Design review of the part built by this model. Coordinates are the model's own, in mm. A direction names the side the tool comes from. Give positions to 0.01 mm unless a question says otherwise; leave off trailing zeros. Loops run counter-clockwise (first coordinate to the right, second up) from the corner with the lowest first, then second, coordinate; pieces in that order, holes last. Notation, with made-up numbers: (57, 50.5) - (68, 50.5) arc R26 ccw to (68, 65.5) - close; hole circle Ø1 at (69, -8). An arc over 180 degrees is marked (long way). Write each question's results on one line, items separated by ' | '.
from build123d import *

# Parameters (mm, degrees)
PAD_DEPTH            = 25
PAD_DEPTH_BACK       = 25
PAD001_START         = 5
PAD001_DEPTH         = 115
PAD002_DEPTH         = 6
PAD002_DEPTH_BACK    = 6
POCKET_DEPTH         = 10.001
POCKET_DEPTH_BACK    = 10.001
POCKET001_DEPTH      = 120.001
PAD003_DEPTH         = 2
LINEARPATTERN_COUNT  = 2
LINEARPATTERN_PITCH  = 8
SKETCH006_W          = 15
SKETCH006_H          = 1
POCKET002_DEPTH      = 7
PAD004_DEPTH         = 6
PAD004_DEPTH_BACK    = 6
SKETCH008_W          = 3.8
SKETCH008_H          = 20
POCKET003_DEPTH      = 60.001
POCKET003_DEPTH_BACK = 60.001
POCKET004_DEPTH      = 10.001
POCKET004_DEPTH_BACK = 10.001


with BuildPart() as part:
    # Sketch → Pad (new body, two sides)
    with BuildSketch(Plane.YZ) as pad_sk:
        Polygon((10, -4.142136), (10, 4.142136), (4.142136, 10), (-4.142136, 10), (-10, 4.142136), (-10, -4.142136), (-4.142136, -10), (4.142136, -10), align=None)
        Polygon((2.5, 1.035534), (1.035534, 2.5), (-1.035534, 2.5), (-2.5, 1.035534), (-2.5, -1.035534), (-1.035534, -2.5), (1.035534, -2.5), (2.5, -1.035534), align=None, mode=Mode.SUBTRACT)
    extrude(amount=PAD_DEPTH)
    extrude(pad_sk.sketch, amount=-PAD_DEPTH_BACK)

    # Sketch001 → Pad001 (join)
    with BuildSketch(Plane.XY.offset(PAD001_START)):
        Polygon((4.5, -1.863961), (4.5, 1.863961), (1.863961, 4.5), (-1.863961, 4.5), (-4.5, 1.863961), (-4.5, -1.863961), (-1.863961, -4.5), (1.863961, -4.5), align=None)
        Polygon((1.575, -0.652386), (1.575, 0.652386), (0.652386, 1.575), (-0.652386, 1.575), (-1.575, 0.652386), (-1.575, -0.652386), (-0.652386, -1.575), (0.652386, -1.575), align=None, mode=Mode.SUBTRACT)
    extrude(amount=PAD001_DEPTH)

    # Sketch002 → Pad002 (join, two sides)
    with BuildSketch(Plane.XZ) as pad002_sk:
        Polygon((-25, 8), (25, 8), (25, 13), (10, 42), (10, 47), (13, 47), (13, 50), (-13, 50), (-13, 47), (-10, 47), (-10, 42), (-25, 13), align=None)
    extrude(amount=PAD002_DEPTH)
    extrude(pad002_sk.sketch, amount=-PAD002_DEPTH_BACK)

    # Sketch003 → Pocket (cut, two sides)
    with BuildSketch(Plane.XZ) as pocket_sk:
        with BuildLine():
            ThreePointArc((7, 8), (0, 15), (-7, 8))
            Line((-7, 8), (7, 8))
        make_face()
    extrude(amount=-POCKET_DEPTH, mode=Mode.SUBTRACT)
    extrude(pocket_sk.sketch, amount=POCKET_DEPTH_BACK, mode=Mode.SUBTRACT)

    # Sketch004 → Pocket001 (cut, through all)
    with BuildSketch(Plane.XY):
        Polygon((1.575, -0.652386), (1.575, 0.652386), (0.652386, 1.575), (-0.652386, 1.575), (-1.575, 0.652386), (-1.575, -0.652386), (-0.652386, -1.575), (0.652386, -1.575), align=None)
    extrude(amount=POCKET001_DEPTH, mode=Mode.SUBTRACT)

    # Sketch005 (on Face68 of Pocket001) → Pad003 (join)
    with BuildSketch(Plane(origin=(0, 0, 120), x_dir=(0, -1, 0), z_dir=(0, 0, 1))):
        Polygon((6.236187, -2.583113), (6.236187, 2.583113), (2.583113, 6.236187), (-2.583113, 6.236187), (-6.236187, 2.583113), (-6.236187, -2.583113), (-2.583113, -6.236187), (2.583113, -6.236187), align=None)
        Polygon((1.339392, -3.233578), (3.233578, -1.339392), (3.233578, 1.339392), (1.339392, 3.233578), (-1.339392, 3.233578), (-3.233578, 1.339392), (-3.233578, -1.339392), (-1.339392, -3.233578), align=None, mode=Mode.SUBTRACT)
    pad003 = extrude(amount=-PAD003_DEPTH)

    # LinearPattern: Pad003 ×2
    with Locations(*[(0, 0, -i * LINEARPATTERN_PITCH) for i in range(1, LINEARPATTERN_COUNT)]):
        add(pad003)

    # Sketch006 (on Face80 of LinearPattern) → Pocket002 (cut)
    with BuildSketch(Plane(origin=(0, 0, 120), x_dir=(0, -1, 0), z_dir=(0, 0, 1))):
        Rectangle(SKETCH006_W, SKETCH006_H)
    extrude(amount=-POCKET002_DEPTH, mode=Mode.SUBTRACT)

    # Sketch007 → Pad004 (join, two sides)
    with BuildSketch(Plane.XZ) as pad004_sk:
        Polygon((-25, -5), (25, -5), (25, -15), (60, -50), (60, -80), (-60, -80), (-60, -50), (-25, -15), align=None)
    extrude(amount=PAD004_DEPTH)
    extrude(pad004_sk.sketch, amount=-PAD004_DEPTH_BACK)

    # Sketch008 → Pocket003 (cut, two sides)
    with BuildSketch(Plane.YZ) as pocket003_sk:
        with Locations((0, -71)):
            Rectangle(SKETCH008_W, SKETCH008_H)
    extrude(amount=-POCKET003_DEPTH, mode=Mode.SUBTRACT)
    extrude(pocket003_sk.sketch, amount=POCKET003_DEPTH_BACK, mode=Mode.SUBTRACT)

    # Sketch009 → Pocket004 (cut, two sides)
    with BuildSketch(Plane.XZ) as pocket004_sk:
        Polygon((-5.142136, -8.142136), (5.142136, -8.142136), (45, -48), (45, -56), (-45, -56), (-45, -48), align=None)
    extrude(amount=-POCKET004_DEPTH, mode=Mode.SUBTRACT)
    extrude(pocket004_sk.sketch, amount=POCKET004_DEPTH_BACK, mode=Mode.SUBTRACT)


solid = part.part
(1) Draft analysis for pull direction X (two halves, no side actions). For faces 1 (the flat face through (-2, 0, 8)), 2 (the flat face through (-60, 3, -65)), 3 (the flat face through (1, 4.5, 115)), state which applies: pulls with the +X half, pulls with the -X half, needs draft (parallel to the pull), parting line crosses it, or undercut.
Answers below:
face 1: undercut | face 2: pulls with the -X half | face 3: needs draft
(2) Take a section at D-D on z = 32. Give the boundary of the cut face in (x, y) (3 decimals).
Answers below:
outline: (-15.172, -6) - (15.172, -6) - (15.172, 6) - (-15.172, 6) - close; hole (-1.575, -0.652) - (-0.652, -1.575) - (0.652, -1.575) - (1.575, -0.652) - (1.575, 0.652) - (0.652, 1.575) - (-0.652, 1.575) - (-1.575, 0.652) - close
(3) Take a section at C-C on x = 18.5. Give the boundary of the cut face in (y, z).
Answers below:
outline: (-10, -4.14) - (-6, -8.14) - (-6, -21.5) - (6, -21.5) - (6, -8.14) - (10, -4.14) - (10, 4.14) - (6, 8.14) - (6, 25.57) - (-6, 25.57) - (-6, 8.14) - (-10, 4.14) - close; (-6, -80) - (-1.9, -80) - (-1.9, -61) - (1.9, -61) - (1.9, -80) - (6, -80) - (6, -56) - (-6, -56) - close; hole (-2.5, -1.04) - (-1.04, -2.5) - (1.04, -2.5) - (2.5, -1.04) - (2.5, 1.04) - (1.04, 2.5) - (-1.04, 2.5) - (-2.5, 1.04) - close
(4) Insertion check: P1, Ø2, axis at x = -1.5, z = 119.5, coming from the +Y side; P2, Ø2, axis at x = -22.5, z = 7.5, coming from the -Y side; P3, Ø1.5, axis at x = 11, y = 7, coming from the -Z side. Each pin has a flat end and moves straight along its axis. Give the tip position at first contact, or say it passes through.
Answers below:
P1: y = 6.24 | P2: y = -7.64 | P3: z = -7.89
(5) Wall thickness on line 1 along Z through (x, y) = (-1.5, 2.75); line 2 along Z through (x, y) = (4.5, -5); line 3 along Z through (x, y) = (4, 0.5): over which ranges is each line inside the solid? List them lowest first. Write a range as from..to.
Answers below:
line 1: -80..-56, -8.14..8, 14.84..120 | line 2: -80..-56, -8.14..8, 13.36..50 | line 3: -61..-56, -8.14..-2.5, 2.5..8, 13.74..120
(6) Take a section at B-B on x = 35. Give the boundary of the cut face in (y, z), plus the area to 3 significant figures.
Answers below:
outline: (-6, -80) - (-1.9, -80) - (-1.9, -61) - (1.9, -61) - (1.9, -80) - (6, -80) - (6, -56) - (-6, -56) - close; (-6, -38) - (6, -38) - (6, -25) - (-6, -25) - close | area: 372 mm2
(7) Tool access review of faces 4 (the flat face through (-10, 0, 45)), 5 (the flat face through (4.44, 4.38, 111.01)), 6 (the flat face through (0.5, -3, 117)), 7 (the flat face through (1, 6, -60)), 8 (the flat face through (45, 0, -52)): name each direction out of +Z, -Z, +X, -X, +Y, -Y from which nothing blocks a thin tool from reaching the whole face with its end or side.
Answers below:
face 4: -X, +Y, -Y | face 5: +Z, +X, +Y | face 6: +Z, +Y, -Y | face 7: -Z, +X, -X, +Y | face 8: +Y, -Y
(8) Take a section at A-A on z = -20.5. Give the boundary of the cut face in (x, y).
Answers below:
outline: (-30.5, -6) - (-17.5, -6) - (-17.5, 6) - (-30.5, 6) - close; (17.5, -6) - (30.5, -6) - (30.5, 6) - (17.5, 6) - close
